Source: CAD feature listing. Evaluate the final solid. Frame: model axes, mm. Face numbers are marked on the shaded views. Round coordinates to 2 decimals unless told otherwise and drop trailing zeros. Write each loop counter-clockwise with the first axis right and the second up, starting at its lowest first coordinate (ties: lowest second). Pieces come first, ordered by that corner, then holes. Notation, with made-up numbers: M 89,4 L 94,4 A12 ccw 94,14 Z; hole C 61.25,0 d3. An arc over 180 degrees is marked long. Answer in a Markdown table with one row per item.
from build123d import *

# Parameters (mm, degrees)
SKETCH1_W           = 73.025
SKETCH1_H           = 73.025
BOSS_EXTRUDE1_DEPTH = 12.7
CHAMFER1_SIZE       = 6.35
SKETCH4_R           = 3.175
CUT_EXTRUDE1_DEPTH  = 3.175
CUT_EXTRUDE2_REACH  = 11.525
SKETCH5_R           = 6.35


with BuildPart() as part:
    # Sketch1 → Boss-Extrude1 (new body)
    with BuildSketch(Plane(origin=(0, 0, 0), x_dir=(1, 0, 0), z_dir=(0, 1, 0))):
        Rectangle(SKETCH1_W, SKETCH1_H)
    extrude(amount=BOSS_EXTRUDE1_DEPTH)

    # Chamfer1
    chamfer1_edges = [part.edges().sort_by_distance(p)[0] for p in [
        (-36.5125, 12.7, 0),
        (0, 12.7, 36.5125),
        (36.5125, 12.7, 0),
        (0, 12.7, -36.5125),
    ]]
    chamfer(chamfer1_edges, length=CHAMFER1_SIZE)

    # Sketch4 → Cut-Extrude1 (cut)
    with BuildSketch(Plane(origin=(0, 12.7, 0), x_dir=(1, 0, 0), z_dir=(0, 1, 0))):
        Circle(SKETCH4_R)
    extrude(amount=-CUT_EXTRUDE1_DEPTH, mode=Mode.SUBTRACT)

    # Sketch5 → Cut-Extrude2 (cut, up to next)
    with BuildSketch(Plane(origin=(0, 9.525, 0), x_dir=(1, 0, 0), z_dir=(0, 1, 0)), mode=Mode.PRIVATE) as cut_extrude2_sk1:
        Circle(SKETCH5_R)
    cut_extrude2_tool1 = extrude(cut_extrude2_sk1.sketch, amount=-CUT_EXTRUDE2_REACH, mode=Mode.PRIVATE) & part.part
    add(cut_extrude2_tool1.solids().sort_by_distance((0, 9.525, 0))[0], mode=Mode.SUBTRACT)


solid = part.part
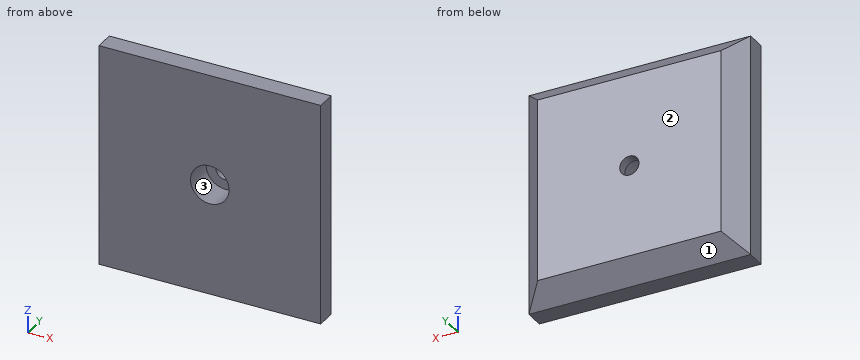
Q1. Section D-D (z = -12). Return loops of the section in (x, y).
Solutions:
| item | result |
|---|---|
| outline | M -36.51,0 L 36.51,0 L 36.51,6.35 L 30.16,12.7 L -30.16,12.7 L -36.51,6.35 Z |
Q2. Contact query for flat-ended pins moving along their axis: pin 1 Ø8.5 at (x, z) = (0, 0) entering from -Y (3 decimals); pin 2 Ø1.5 at (x, y) = (1, 9) entering from -Z. Output: stop coordinate, or through.
Solutions:
| item | result |
|---|---|
| pin 1 | stops at y = 9.525 |
| pin 2 | stops at z = -34.61 |
Q3. Material intervals for probe 1 along Z at (x, y) = (0, 6); probe 2 along X at (y, z) = (10.75, 0) (1 decimal), sorted ascending.
Solutions:
| item | result |
|---|---|
| probe 1 | z = -36.51 to -6.35, 6.35 to 36.51 |
| probe 2 | x = -32.1 to -3.2, 3.2 to 32.1 |
Q4. Section C-C (y = 2). Return loops of the section in (x, z), and give its area (3 significant figures).
Solutions:
| item | result |
|---|---|
| outline | M -36.51,-36.51 L 36.51,-36.51 L 36.51,36.51 L -36.51,36.51 Z; hole C 0,0 d12.7 |
| area | 5,210 mm2 |
Q5. Pull-direction query (Z, two-part tool) for the marked faces 1, 2 and 3; classes: pulls with the +Z half, pulls with the -Z half, needs draft (parallel to the pull), parting line crosses it, or undercut.
Solutions:
| item | result |
|---|---|
| face 1 | pulls with the -Z half |
| face 2 | needs draft |
| face 3 | undercut |
